from build123d import *

# Parameters (mm, degrees)
F0_W        = 80.0557104707
F0_H        = 80.0557104707
F0_W_2      = 73.7057104707
F0_H_2      = 73.7057104707
F0_W_3      = 39.99992
F0_H_3      = 39.99992
F1_DEPTH    = 6.35
F2_DEPTH    = 9.144
F3_DEPTH    = 139.7
F4_W        = 20.0278952353
F4_H        = 3.175
F5_DEPTH    = 3.175
F7_SIZE     = 5.08
F6_T1_DEPTH = 177.6130734528


# Not quite as in the source:
# - a fillet or chamfer that OpenCascade refuses, or shapes differently, is made with other operations: its cross-section is extruded or revolved along the edge and cut away or added


with BuildPart() as f1:
    # F0 (on Top) → F1 (new body)
    with BuildSketch(Plane.XY):
        Rectangle(F0_W, F0_H)
        Rectangle(F0_W_2, F0_H_2, mode=Mode.SUBTRACT)
        Rectangle(F0_W_2, F0_H_2)
        Rectangle(F0_W_3, F0_H_3, mode=Mode.SUBTRACT)
        Rectangle(F0_W_3, F0_H_3)
    extrude(amount=-F1_DEPTH)

    # F0 (on Top) → F2 (cut)
    with BuildSketch(Plane.XY):
        Rectangle(F0_W_3, F0_H_3)
    extrude(amount=-F2_DEPTH, mode=Mode.SUBTRACT)

    # F0 (on Top) → F3 (join)
    with BuildSketch(Plane.XY):
        Rectangle(F0_W, F0_H)
        Rectangle(F0_W_2, F0_H_2, mode=Mode.SUBTRACT)
    extrude(amount=F3_DEPTH)

    # F4 (on face) → F5 (cut)
    with BuildSketch(Plane(origin=(0, 0, -6.35), x_dir=(1, 0, 0), z_dir=(0, 0, -1))):
        with Locations((30.0139076177, 18.41246)):
            Rectangle(F4_W, F4_H)
        with Locations((30.0139076177, -18.41246)):
            Rectangle(F4_W, F4_H)
    extrude(amount=-F5_DEPTH, mode=Mode.SUBTRACT)

    # F7
    f7_edges = [f1.edges().sort_by_distance(p)[0] for p in [
        (40.027855, -40.027855, 66.675),
        (-40.027855, -40.027855, 66.675),
        (-40.027855, 40.027855, 66.675),
        (40.027855, 40.027855, 66.675),
    ]]
    chamfer(f7_edges, length=F7_SIZE)

    # F6: fillet of radius 15.24 on 8 edges, made by hand

    # F6_s2 → F6_t1 (cut)
    with BuildSketch(Plane.XY.offset(-22.1315367264)):
        with BuildLine():
            ThreePointArc((-28.6352405448, -40.0278552353), (-34.467336054, -38.8677793108), (-39.4115478901, -35.5641625806))
            Line((-39.4115478901, -35.5641625806), (-34.9478552353, -40.0278552353))
            Line((-34.9478552353, -40.0278552353), (-28.6352405448, -40.0278552353))
        make_face()
        with BuildLine():
            ThreePointArc((-35.5641625806, -39.4115478901), (-38.8677793108, -34.467336054), (-40.0278552353, -28.6352405448))
            Line((-40.0278552353, -28.6352405448), (-40.0278552353, -34.9478552353))
            Line((-40.0278552353, -34.9478552353), (-35.5641625806, -39.4115478901))
        make_face()
        with BuildLine():
            ThreePointArc((-35.5641625806, 39.4115478901), (-38.8677793108, 34.467336054), (-40.0278552353, 28.6352405448))
            Line((-40.0278552353, 28.6352405448), (-40.0278552353, 34.9478552353))
            Line((-40.0278552353, 34.9478552353), (-35.5641625806, 39.4115478901))
        make_face()
        with BuildLine():
            ThreePointArc((-28.6352405448, 40.0278552353), (-34.467336054, 38.8677793108), (-39.4115478901, 35.5641625806))
            Line((-39.4115478901, 35.5641625806), (-34.9478552353, 40.0278552353))
            Line((-34.9478552353, 40.0278552353), (-28.6352405448, 40.0278552353))
        make_face()
        with BuildLine():
            ThreePointArc((40.0278552353, -28.6352405448), (38.8677793108, -34.467336054), (35.5641625806, -39.4115478901))
            Line((35.5641625806, -39.4115478901), (40.0278552353, -34.9478552353))
            Line((40.0278552353, -34.9478552353), (40.0278552353, -28.6352405448))
        make_face()
        with BuildLine():
            ThreePointArc((39.4115478901, -35.5641625806), (34.467336054, -38.8677793108), (28.6352405448, -40.0278552353))
            Line((28.6352405448, -40.0278552353), (34.9478552353, -40.0278552353))
            Line((34.9478552353, -40.0278552353), (39.4115478901, -35.5641625806))
        make_face()
        with BuildLine():
            ThreePointArc((40.0278552353, 28.6352405448), (38.8677793108, 34.467336054), (35.5641625806, 39.4115478901))
            Line((35.5641625806, 39.4115478901), (40.0278552353, 34.9478552353))
            Line((40.0278552353, 34.9478552353), (40.0278552353, 28.6352405448))
        make_face()
        with BuildLine():
            ThreePointArc((39.4115478901, 35.5641625806), (34.467336054, 38.8677793108), (28.6352405448, 40.0278552353))
            Line((28.6352405448, 40.0278552353), (34.9478552353, 40.0278552353))
            Line((34.9478552353, 40.0278552353), (39.4115478901, 35.5641625806))
        make_face()
    extrude(amount=F6_T1_DEPTH, mode=Mode.SUBTRACT)


solid = f1.part
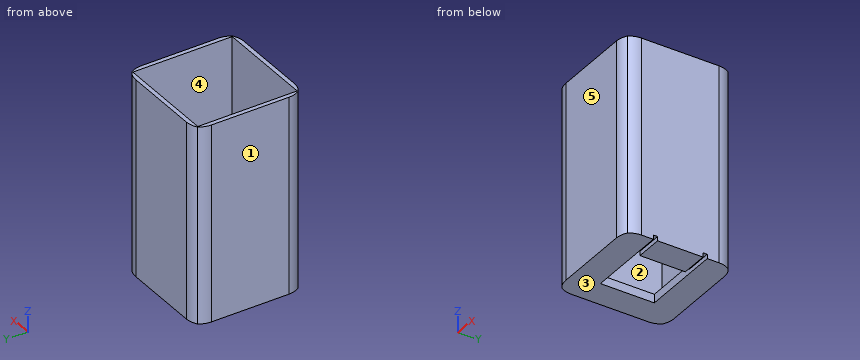
Verification items for the finished model (mm, model axes). Face numbers are marked on the shaded views. A direction names the side the tool comes from. Round coordinates to 2 decimals unless told otherwise and drop trailing zeros. Write each loop counter-clockwise with the first axis right and the second up, starting at its lowest first coordinate (ties: lowest second). Pieces come first, ordered by that corner, then holes.
(1) Section check B-B (z = 108.5). Enter the section's corners in (x, y).
Returned:
outline: (-40.03, -28.64) arc R15.24 ccw to (-37.31, -37.31) arc R15.24 ccw to (-28.64, -40.03) - (28.64, -40.03) arc R15.24 ccw to (37.31, -37.31) arc R15.24 ccw to (40.03, -28.64) - (40.03, 28.64) arc R15.24 ccw to (37.31, 37.31) arc R15.24 ccw to (28.64, 40.03) - (-28.64, 40.03) arc R15.24 ccw to (-37.31, 37.31) arc R15.24 ccw to (-40.03, 28.64) - close; hole (-36.85, -36.85) - (36.85, -36.85) - (36.85, 36.85) - (-36.85, 36.85) - close
(2) Access from +Z, -Z, +X, -X, +Y, -Y to the whole of each face (thin tool, end or side, straight path). Record for the marked faces 4 and 5.
Returned:
face 4: +Z
face 5: +Z, -Z, +X, -X, -Y
(3) Section check A-A (x = 0.5). Enter the section's corners in (y, z), plus the area to 3 significant figures.
Returned:
outline: (-40.03, -6.35) - (-20, -6.35) - (-20, 0) - (-36.85, 0) - (-36.85, 139.7) - (-40.03, 139.7) - close; (20, -6.35) - (40.03, -6.35) - (40.03, 139.7) - (36.85, 139.7) - (36.85, 0) - (20, 0) - close
area: 1,140 mm2
(4) Material ranges on line 1 (Y direction, x = -27.5, z = 111); line 2 (Z direction, x = 20, y = 32.5), recorded low to high.
Returned:
line 1: y = -40.03 to -36.85, 36.85 to 40.03
line 2: z = -6.35 to 0
(5) Section check D-D (x = 22). Enter the section's corners in (y, z) (3 decimals), plus the area to 3 significant figures.
Returned:
outline: (-40.028, -6.35) - (-20, -6.35) - (-20, -3.175) - (-16.825, -3.175) - (-16.825, -6.35) - (16.825, -6.35) - (16.825, -3.175) - (20, -3.175) - (20, -6.35) - (40.028, -6.35) - (40.028, 139.7) - (36.853, 139.7) - (36.853, 0) - (-36.853, 0) - (-36.853, 139.7) - (-40.028, 139.7) - close
area: 1,380 mm2
(6) Mould release check, pull along X, two halves, no side actions. Record for the marked faces 1, 2 and 3: pulls with the +X half, pulls with the -X half, needs draft (parallel to the pull), parting line crosses it, or undercut.
Returned:
face 1: pulls with the -X half
face 2: undercut
face 3: needs draft
(7) Depth check by flat-ended pin: pin 1 Ø2.5 at (x, z) = (30.5, -5.5) entering from +Y; pin 2 Ø1.6 at (x, y) = (32, -18) entering from -Z (3 decimals). Enter the tip coordinate at first touch or a pass-through.
Returned:
pin 1: stops at y = 40.02
pin 2: stops at z = -3.175
